CAD build for the part. Positions are in the model's coordinates, mm. Coordinates: 2 decimals unless noted, no trailing zeros. Write each loop counter-clockwise with the first axis right and the second up, starting at its lowest first coordinate (ties: lowest second). Pieces come first, ordered by that corner, then holes. Notation, with made-up numbers: (-1.5, 89.5) - (42.5, 89.5) arc R18 cw to (42.5, 124.5) - close; hole circle Ø11 at (41, 56). An arc over 180 degrees is marked (long way). One line per question, with ' | ' between items. Start each with the question number.
1. Probe line 1 (Y direction, x = -3.5, z = -0.2); line 2 (Y direction, x = -27, z = -0.55); line 3 (X direction, y = -20, z = -0.25). List the from-to ranges inside material, lowest first.
2. Band-saw the part on A-A, the plane x = 13. Write the cut outline in (y, z), then the cut area to 3 significant figures.
3. Band-saw the part on B-B, the plane z = -0.35. Write the cut outline in (x, y).
Autodesk Fusion 360 part; units mm, degrees
sketch "LED window" plane through (0, 0, 0) normal (0, 0, 1) x (1, 0, 0)
  line L0 (23.6586, 17.7446) -> (-28.2697, 17.7446)
  line L1 (-28.2697, 17.7446) -> (-28.2697, -2.7419)
  line L2 (-28.2697, -2.7419) -> (23.6586, -2.7419)
  line L3 (23.6586, -2.7419) -> (23.6586, 17.7446)
sketch "Bottom" plane through (0, 0, 0) normal (0, 0, 1) x (1, 0, 0)
  line L0 (-37.1804, -23.3607) -> (36.4196, -23.3607)
  line L1 (36.4196, -23.3607) -> (36.4196, 26.1393)
  line L2 (36.4196, 26.1393) -> (-37.1804, 26.1393)
  line L3 (-37.1804, 26.1393) -> (-37.1804, -23.3607)
  dimension "d148" = 73.6
  dimension "d149" = 49.5
extrude "Extrude32" add sketch "Bottom" along normal blind 1.5 draft -45 makes body 1
ref_plane "WorkPlane3" through (-37.1804, 1.3893, 0) normal (1, 0, 0) x (0, -1, 0)
sketch "Sketch23" plane through (-37.1804, -58.3607, 0) normal (1, 0, 0) x (0, 1, 0)
  line L0 (84.5, 0) -> (35, 0)
  line L1 (35, 0) -> (35, 1.5002)
  line L2 (35, 1.5002) -> (84.5, 1.5002)
  line L3 (84.5, 1.5002) -> (84.5, 0)
  line L4 (35, 0) -> (36.5005, 1.5002)
  line L5 (82.9998, 1.5002) -> (84.5, 1.5002)
  line L6 (82.9998, 1.5002) -> (84.5, 0)
  line L7 (84.5, 0) -> (84.5, 1.5002)
  point P0 (84.5, 0)
  dimension "d167" = 49.5
extrude "Extrude33" add sketch "Sketch23" along normal blind 1 contours L0 L2 L4 L6 bodies 1
extrude "Extrude34" add 1 faces at (-36.1804, -6.3605, 1.1667) along direction (1, 0, 0) blind 1.4 on bodies 1 bodies 1
mirror "Mirror1" about plane through (0, 0, 0) normal (0, 0, 1) of bodies 1 makes body 2
hidden bodies 1
equation "WALL = 18.5 mm + TOP_H"
equation "WALL_THICK = TOP_H"
equation "OUTER_HEIGHT = 6.4 mm + TOP_H"
equation "INNER_HEIGHT = OUTER_HEIGHT + 3.5 mm"
equation "d148 = TOP_WIDTH - ( WALL_THICK * 2 ) + 1.1 mm"
equation "d149 = TOP_HEIGHT - WALL_THICK * 2 - 0.5 mm"
equation "d150 = WALL_THICK"
equation "d167 = TOP_HEIGHT - WALL_THICK * 2 - 0.5 mm"
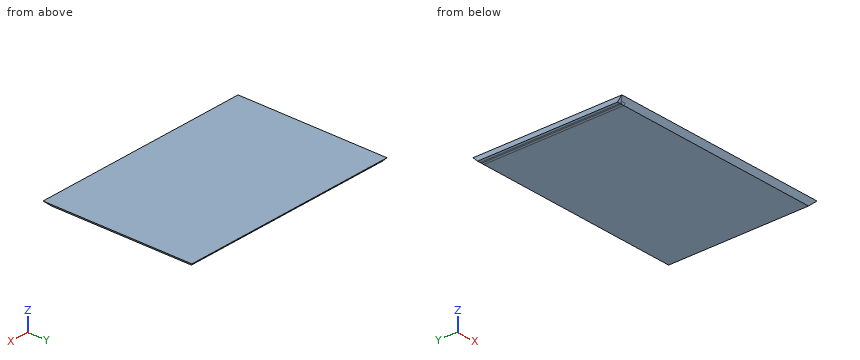
Filled in:
1) line 1: y = -23.16 to 25.94 | line 2: y = -22.81 to 25.59 | line 3: x = -37.18 to 36.17
2) outline: (-23.36, 0) - (-21.86, -1.5) - (24.64, -1.5) - (26.14, 0) - close | area: 72.0 mm²
3) outline: (-37.18, -23.01) - (36.07, -23.01) - (36.07, 25.79) - (-37.18, 25.79) - close
